from build123d import *

# Parameters (mm, degrees)
SKETCH1_R             = 52.5
SKETCH1_R_2           = 42.5
BOSS_EXTRUDE1_DEPTH   = 25
SKETCH1_R_3           = 21.666666667
SKETCH1_R_4           = 11.666666667
BOSS_EXTRUDE1_2_DEPTH = 25
BOSS_EXTRUDE1_3_DEPTH = 25
SKETCH2_R             = 52.5
SKETCH2_R_2           = 42.5
BOSS_EXTRUDE2_DEPTH   = 38
BOSS_EXTRUDE3_DEPTH   = 11
CUT_EXTRUDE1_DEPTH    = 2


with BuildPart() as part:
    # Sketch1 → Boss-Extrude1 (new body)
    with BuildSketch(Plane(origin=(0, 0, 0), x_dir=(0, 0, -1), z_dir=(1, 0, 0))):
        Circle(SKETCH1_R)
        Circle(SKETCH1_R_2, mode=Mode.SUBTRACT)
    extrude(amount=BOSS_EXTRUDE1_DEPTH)

    # Sketch2 → Boss-Extrude2 (add)
    with BuildSketch(Plane(origin=(25, 0, 0), x_dir=(0, 0, -1), z_dir=(1, 0, 0))):
        Circle(SKETCH2_R)
        Circle(SKETCH2_R_2, mode=Mode.SUBTRACT)
    extrude(amount=BOSS_EXTRUDE2_DEPTH)



with BuildPart() as body_2:
    # Sketch1 → Boss-Extrude1 2 (new body)
    with BuildSketch(Plane(origin=(0, 0, 0), x_dir=(0, 0, -1), z_dir=(1, 0, 0))):
        with Locations((87.5, 0)):
            Circle(SKETCH1_R_3)
        with Locations((87.5, 0)):
            Circle(SKETCH1_R_4, mode=Mode.SUBTRACT)
    extrude(amount=BOSS_EXTRUDE1_2_DEPTH)


with BuildPart() as body_3:
    # Sketch1 → Boss-Extrude1 3 (new body)
    with BuildSketch(Plane(origin=(0, 0, 0), x_dir=(0, 0, -1), z_dir=(1, 0, 0))):
        with Locations((-87.5, 0)):
            Circle(SKETCH1_R_3)
        with Locations((-87.5, 0)):
            Circle(SKETCH1_R_4, mode=Mode.SUBTRACT)
    extrude(amount=BOSS_EXTRUDE1_3_DEPTH)


with BuildPart() as part_1:
    add(part.part)

    add(body_2.part)  # Boss-Extrude3 merges body 2

    add(body_3.part)  # Boss-Extrude3 merges body 3
    # Sketch4 → Boss-Extrude3 (add)
    with BuildSketch(Plane(origin=(0, 0, 0), x_dir=(0, 0, -1), z_dir=(1, 0, 0))):
        with BuildLine():
            Line((18.5, 49.132473986), (95.134920635, 20.276894026))
            ThreePointArc((95.134920635, 20.276894026), (65.833333333, 0), (95.134920635, -20.276894026))
            Line((95.134920635, -20.276894026), (18.5, -49.132473986))
            ThreePointArc((18.5, -49.132473986), (52.5, 0), (18.5, 49.132473986))
        make_face()
        with BuildLine():
            Line((-95.134920635, -20.276894026), (-18.5, -49.132473986))
            ThreePointArc((-18.5, -49.132473986), (-52.5, 0), (-18.5, 49.132473986))
            Line((-18.5, 49.132473986), (-95.134920635, 20.276894026))
            ThreePointArc((-95.134920635, 20.276894026), (-65.833333333, 0), (-95.134920635, -20.276894026))
        make_face()
    extrude(amount=BOSS_EXTRUDE3_DEPTH)

    # Sketch5 → Cut-Extrude1 (cut)
    with BuildSketch(Plane(origin=(11, 0, 0), x_dir=(0, 0, -1), z_dir=(1, 0, 0))):
        with BuildLine():
            Line((-77.005456237, -24.966157006), (-44.91894061, -37.047790413))
            ThreePointArc((-44.91894061, -37.047790413), (-42.59745711, -36.353451861), (-42.649075034, -33.930906247))
            ThreePointArc((-42.649075034, -33.930906247), (-54.5, 0), (-42.649075034, 33.930906247))
            ThreePointArc((-42.649075034, 33.930906247), (-42.59745711, 36.353451861), (-44.91894061, 37.047790413))
            Line((-44.91894061, 37.047790413), (-77.005456237, 24.966157006))
            ThreePointArc((-77.005456237, 24.966157006), (-78.298605787, 23.185821053), (-77.173367501, 21.294876669))
            ThreePointArc((-77.173367501, 21.294876669), (-63.833333333, 0), (-77.173367501, -21.294876669))
            ThreePointArc((-77.173367501, -21.294876669), (-78.298605787, -23.185821053), (-77.005456237, -24.966157006))
        make_face()
        with BuildLine():
            Line((77.005456237, 24.966157006), (44.91894061, 37.047790413))
            ThreePointArc((44.91894061, 37.047790413), (42.59745711, 36.353451861), (42.649075034, 33.930906247))
            ThreePointArc((42.649075034, 33.930906247), (54.5, 0), (42.649075034, -33.930906247))
            ThreePointArc((42.649075034, -33.930906247), (42.59745711, -36.353451861), (44.91894061, -37.047790413))
            Line((44.91894061, -37.047790413), (77.005456237, -24.966157006))
            ThreePointArc((77.005456237, -24.966157006), (78.298605787, -23.185821053), (77.173367501, -21.294876669))
            ThreePointArc((77.173367501, -21.294876669), (63.833333333, 0), (77.173367501, 21.294876669))
            ThreePointArc((77.173367501, 21.294876669), (78.298605787, 23.185821053), (77.005456237, 24.966157006))
        make_face()
    extrude(amount=-CUT_EXTRUDE1_DEPTH, mode=Mode.SUBTRACT)


solid = part_1.part
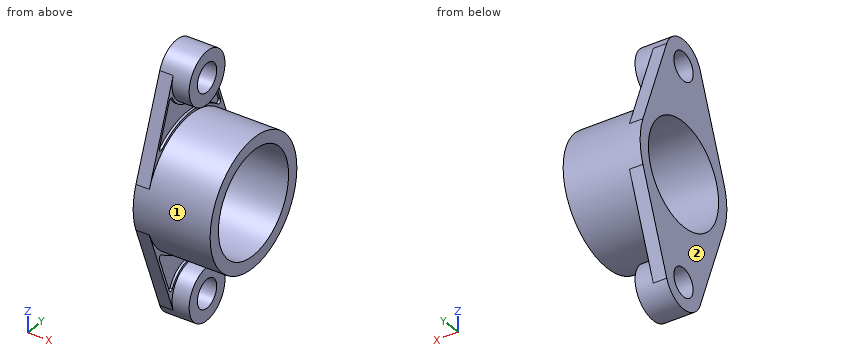
Design review of the part built by this model. Coordinates are the model's own, in mm. Face numbers are marked on the shaded views. A direction names the side the tool comes from. Round coordinates to 2 decimals unless told otherwise and drop trailing zeros. Write each loop counter-clockwise with the first axis right and the second up, starting at its lowest first coordinate (ties: lowest second). Pieces come first, ordered by that corner, then holes.
Item 1: For the marked faces 1 and 2, list the 3-axis set-ups (+Z, -Z, +X, -X, +Y, -Y) from which the entire face can be reached by the end or side of a thin tool; tool diameter is ignored.
Item 2: For pin 1 Ø2 at (x, y) = (47, 5.5) entering from +Z; pin 2 Ø18.5 at (y, z) = (0, 87.5) entering from -X; pin 3 Ø21.5 at (y, z) = (4.5, -89.5) entering from +X; pin 4 Ø1 at (x, z) = (10.5, 76) entering from -Y, all flat-tipped, find the tip position at first contact; note any pin that passes through.
Item 3: Consider section C-C on y = -29. Give the boundary of the cut face in (x, z).
Item 4: Wall thickness on L1, parallel to Y at x = 15, z = 0; L2, parallel to X at y = -5, z = -56.5; L3, parallel to Z at x = 54, y = 5: over which ranges is each line inside the solid? List them lowest first.
Item 5: Consider section A-A on y = 0. Count the separate pieces of the cut face and the enclosed holes in it, and give its area (3 significant figures).
Item 6: Consider section B-B on z = -14.5. Give the boundary of the cut face in (x, y), and give its area (3 significant figures).
Item 7: Consider section D-D on z = -73.5. Give the boundary of the cut face in (x, y).
Check values:
1. face 1: +X
1. face 2: +Z, -Z, -X, +Y, -Y
2. pin 1: stops at z = 52.31
2. pin 2: passes through
2. pin 3: stops at x = 25
2. pin 4: stops at y = -27.67
3. outline: (0, -71.97) - (11, -71.97) - (11, -66.29) - (9, -66.29) - (9, -46.14) - (11, -46.14) - (11, -43.76) - (63, -43.76) - (63, -31.07) - (0, -31.07) - close; (0, 31.07) - (63, 31.07) - (63, 43.76) - (11, 43.76) - (11, 46.14) - (9, 46.14) - (9, 66.29) - (11, 66.29) - (11, 71.97) - (0, 71.97) - close
4. L1: y = -52.5 to -42.5, 42.5 to 52.5
4. L2: x = 0 to 9
4. L3: z = -52.26 to -42.2, 42.2 to 52.26
5. separate pieces: 4
5. enclosed holes: 0
5. area: 2,520 mm2
6. outline: (0, -50.46) - (63, -50.46) - (63, -39.95) - (0, -39.95) - close; (0, 39.95) - (63, 39.95) - (63, 50.46) - (0, 50.46) - close
6. area: 1,320 mm2
7. outline: (0, -28.42) - (11, -28.42) - (11, -26.29) - (9, -26.29) - (9, -19.08) - (11, -19.08) - (11, -16.54) - (25, -16.54) - (25, 16.54) - (11, 16.54) - (11, 19.08) - (9, 19.08) - (9, 26.29) - (11, 26.29) - (11, 28.42) - (0, 28.42) - close
